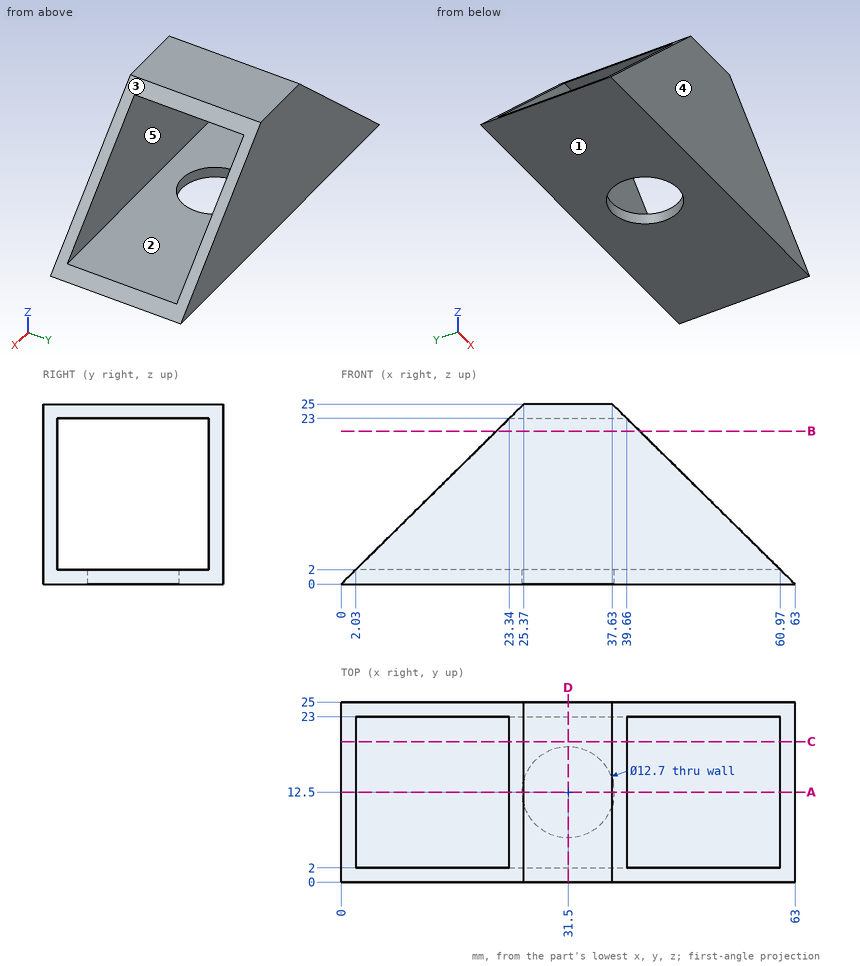
Geometry: see drawing. Coordinates: mm, zero at the bounding-box minimum. A direction names the side the tool comes from. Coordinates: 2 decimals unless noted, no trailing zeros. Loops run counter-clockwise (first coordinate to the right, second up) from the corner with the lowest first, then second, coordinate; pieces in that order, holes last. Notation, with made-up numbers: (-22, 49.25) -> (21, 49.25) arc R20 ccw to (21, 64.25) -> close; hole circle Ø10 at (-15, 88.5). An arc over 180 degrees is marked (long way). Write item = value, one per line. Start each with the question number.
Item 1: Reachability of the marked faces 4 and 5 from +Z, -Z, +X, -X, +Y, -Y: full face, straight path, thin tool, end or side. Return the list, or none.
Item 2: Cut plane A-A, the plane y = 12.5. Return loops of the section in (x, z), plus the area to 3 significant figures.
Item 3: Cut plane D-D, the plane x = 31.5. Return loops of the section in (y, z).
Item 4: Mould query, pull axis Z, two halves, no side actions, for the marked faces 1, 2 and 3. Classes: pulls with the +Z half, pulls with the -Z half, needs draft (parallel to the pull), parting line crosses it, or undercut.
Item 5: Material intervals for line 1 (Y direction, x = 31.5, z = 0.7); line 2 (Z direction, x = 29, y = 6), sorted ascending.
Item 6: Cut plane B-B, the plane z = 21.25. Return loops of the section in (x, y) (1 decimal).
Item 7: Cut plane C-C, the plane y = 19.5. Return loops of the section in (x, z).
Item 8: First-contact query: P1, Ø6, axis at x = 31.5, y = 14.5, coming from the -Z side; P2, Ø2, axis at x = 19, y = 3.5, coming from the +Z side. Flat tips, straight axial feed; report the tip coordinate or a pass-through.
Ans:
q1.face_4 = +Z, -Z, +X, -X, -Y
q1.face_5 = +X, -X
q2.outline = (0, 0) -> (25.15, 0) -> (25.15, 2) -> (2.03, 2) -> close; (23.34, 23) -> (39.66, 23) -> (37.63, 25) -> (25.37, 25) -> close; (37.85, 0) -> (63, 0) -> (60.97, 2) -> (37.85, 2) -> close
q2.area = 125 mm²
q3.outline = (0, 0) -> (6.15, 0) -> (6.15, 2) -> (2, 2) -> (2, 23) -> (23, 23) -> (23, 2) -> (18.85, 2) -> (18.85, 0) -> (25, 0) -> (25, 25) -> (0, 25) -> close
q4.face_1 = pulls with the -Z half
q4.face_2 = undercut
q4.face_3 = pulls with the +Z half
q5.line_1 = 0 to 6.15, 18.85 to 25
q5.line_2 = 0 to 2, 23 to 25
q6.outline = (21.6, 0) -> (41.4, 0) -> (41.4, 2) -> (21.6, 2) -> close; (21.6, 23) -> (41.4, 23) -> (41.4, 25) -> (21.6, 25) -> close
q7.outline = (0, 0) -> (63, 0) -> (60.97, 2) -> (2.03, 2) -> close; (23.34, 23) -> (39.66, 23) -> (37.63, 25) -> (25.37, 25) -> close
q8.P1 = 23
q8.P2 = 2
